Solid Edge part; units mm, degrees
sketch "Sketch1" plane through (0, 0, 0) normal (0, -1, 0) x (1, 0, 0)
  line L0 (33.7037, 66.6239) -> (103.7037, 66.6239)
  line L1 (103.7037, 66.6239) -> (103.7037, 26.6239)
  line L2 (103.7037, 26.6239) -> (33.7037, 26.6239)
  line L3 (33.7037, 26.6239) -> (33.7037, 66.6239)
  dimension "D1" = 33.7037
  dimension "D2" = 103.7037
  dimension "D3" = 103.7037
  dimension "D4" = 33.7037
extrude "Protrusion1" add sketch "Sketch1" against normal blind 15
sketch "Sketch2" plane through (68.7037, 0, 46.6239) normal (0, -1, 0) x (1, 0, 0)
  circle A0 centre (0, 10) radius 5.5
extrude "ExtrudedCutout_1" cut sketch "Sketch2" against normal blind 12
sketch "Sketch3" plane through (103.7037, 7.5, 46.6239) normal (1, 0, 0) x (0, 1, 0)
  line L0 (-7.5, 12.6) -> (-1.5, 12.6)
  arc A0 (-1.5, 12.6) -> (-1.5, 7.4) centre (-1.5, 10) cw
  line L1 (-1.5, 7.4) -> (-7.5, 7.4)
  line L2 (-7.5, 7.4) -> (-7.5, 12.6)
  dimension "D1" = 7.5
extrude "ExtrudedCutout_4" cut sketch "Sketch3" against normal blind 15
sketch "Sketch4" plane through (88.7037, 4.3, 55.6239) normal (1, 0, 0) x (0, 1, 0)
  line L0 (-4.3, 6) -> (1.7, 6)
  arc A0 (1.7, 6) -> (1.7, -5) centre (1.7, 0.5) cw
  line L1 (1.7, -5) -> (-4.3, -5)
  line L2 (-4.3, -5) -> (-4.3, 6)
  dimension "D1" = 4.3
extrude "ExtrudedCutout_5" cut sketch "Sketch4" against normal blind 15
sketch "Sketch5" plane through (33.7037, 7.5, 46.6239) normal (-1, 0, 0) x (0, -1, 0)
  line L0 (7.5, 12.6) -> (1.5, 12.6)
  arc A0 (1.5, 12.6) -> (1.5, 7.4) centre (1.5, 10) ccw
  line L1 (1.5, 7.4) -> (7.5, 7.4)
  line L2 (7.5, 7.4) -> (7.5, 12.6)
  dimension "D1" = 7.5
  dimension "D2" = 7.5
extrude "ExtrudedCutout_6" cut sketch "Sketch5" against normal blind 15
sketch "Sketch6" plane through (48.7037, 4.3, 56.6239) normal (-1, 0, 0) x (0, -1, 0)
  line L0 (4.3, 5.5) -> (-1.7, 5.5)
  arc A0 (-1.7, 5.5) -> (-1.7, -5.5) centre (-1.7, 0) ccw
  line L1 (-1.7, -5.5) -> (4.3, -5.5)
  line L2 (4.3, -5.5) -> (4.3, 5.5)
  dimension "D1" = 4.3
  dimension "D2" = 4.3
extrude "ExtrudedCutout_7" cut sketch "Sketch6" against normal blind 9
sketch "Sketch7" plane through (57.7037, 5.75, 56.6239) normal (-1, 0, 0) x (0, -1, 0)
  line L0 (5.75, 3.9) -> (-0.25, 3.9)
  arc A0 (-0.25, 3.9) -> (-0.0606, -4.0955) centre (-0.25, -0.1) ccw
  line L1 (-0.0606, -4.0955) -> (5.75, -4.0955)
  line L2 (5.75, -4.0955) -> (5.75, 3.9)
  dimension "D1" = 5.75
  dimension "D2" = 5.75
extrude "Cutout1" cut sketch "Sketch7" against normal up to next
sketch "Sketch8" plane through (68.7037, 7.5, 26.6239) normal (0, 0, -1) x (1, 0, 0)
  line L0 (-6, 7.5) -> (-6, 1.5)
  arc A0 (-6, 1.5) -> (6, 1.5) centre (0, 1.5) ccw
  line L1 (6, 1.5) -> (6, 7.5)
  line L2 (6, 7.5) -> (-6, 7.5)
  dimension "D1" = 6
extrude "ExtrudedCutout_9" cut sketch "Sketch8" against normal blind 15
sketch "Sketch9" plane through (68.7037, 5.75, 41.6239) normal (0, 0, -1) x (1, 0, 0)
  line L0 (-3.4391, 5.75) -> (-3.4391, -0.25)
  arc A0 (-3.4391, -0.25) -> (4.5609, -0.25) centre (0.5609, -0.25) ccw
  line L1 (4.5609, -0.25) -> (4.5609, 5.75)
  line L2 (4.5609, 5.75) -> (-3.4391, 5.75)
  dimension "D1" = 3.4391
extrude "Cutout2" cut sketch "Sketch9" against normal up to next
Can you work these out from the model? Positions are in its coordinate system, mm. A direction names the side the tool comes from. Coordinates: 2 decimals unless noted, no trailing zeros. Write each loop counter-clockwise with the first axis right and the second up, starting at its lowest first coordinate (ties: lowest second). Pieces come first, ordered by that corner, then holes.
Q1. If we mould it in two halves opening along X, with no side actions, what happens to faces 5 (the face through (68.6, 12, 34)), 6 (the face through (103.704, 7, 47)), 7 (the face through (33.704, 7, 46))? For each: +X half, -X half, draft (parallel to the pull), parting line (faces both ways), or undercut.
Results found:
face 5: undercut
face 6: +X half
face 7: -X half
Q2. Imagine slicing it at A-A, the plane y = 2.75. Count the separate pieces of the cut face and the enclosed holes in it, plus the area to 3 significant figures.
Results found:
separate pieces: 3
enclosed holes: 0
area: 1,980 mm2
Q3. Imagine slicing it at C-C, the plane x = 84. List the corners of the cut face in (y, z) for me.
Results found:
outline: (0, 26.62) - (15, 26.62) - (15, 66.62) - (0, 66.62) - (0, 61.62) - (6, 61.62) arc R5.5 cw to (6, 50.62) - (0, 50.62) - close
Q4. For P1, Ø3.5, axis at y = 5, z = 56.5, coming from the -X side; P2, Ø6, axis at x = 66, y = 5, coming from the -Z side, each with a flat end and sliding along its axis, tell me the tip position at first contact or that it passes through.
Results found:
P1: passes through
P2: stops at z = 41.62
Q5. Please list where these lines run through material, in increasing order: L1, parallel to Z at x = 77, y = 1.25; L2, parallel to X at y = 7.5, z = 52.5; L3, parallel to X at y = 1.5, z = 47.5.
Results found:
L1: z = 26.62 to 50.62, 61.62 to 66.62
L2: x = 33.7 to 48.7, 57.7 to 65.06, 72.97 to 73.7, 88.7 to 103.7
L3: x = 33.7 to 65.26, 73.26 to 103.7
Q6. Which directions (+Z, -Z, +X, -X, +Y, -Y) give clear straight access to the entire face, cutting with the end or side of a thin tool? Please do faces 1 (the face through (96, 3, 54.024)), 2 (the face through (48.704, 8, 59)), 3 (the face through (65.265, 3, 47)), 4 (the face through (69, 15, 46)).
Results found:
face 1: +X, -Y
face 2: -Y
face 3: -Z, -Y
face 4: +Z, -Z, +X, -X, +Y
Q7. Imagine slicing it at B-B, the plane z = 33. List the corners of the cut face in (x, y) for me.
Results found:
outline: (33.7, 0) - (62.7, 0) - (62.7, 6) arc R6 cw to (74.7, 6) - (74.7, 0) - (103.7, 0) - (103.7, 15) - (33.7, 15) - close
